Build history of the part. All positions in model axes, mm. Face numbers are marked on the shaded views. Round coordinates to 2 decimals unless told otherwise and drop trailing zeros. Write each loop counter-clockwise with the first axis right and the second up, starting at its lowest first coordinate (ties: lowest second). Pieces come first, ordered by that corner, then holes. Notation, with made-up numbers: (-32.5, -17) - (-7.5, -17) arc R15 cw to (-7.5, -1) - close; hole circle Ø7 at (30, 3). An arc over 180 degrees is marked (long way). One line per question, with ' | ' between items.
from build123d import *

# Parameters (mm, degrees)
SKETCH1_W                = 46
SKETCH1_H                = 12
BOSS_EXTRUDE1_DEPTH      = 12
F_7_0_7_DIAMETER_HOLE1_D = 7
M6X1_0_TAPPED_HOLE1_D    = 5


with BuildPart() as part:
    # Sketch1 → Boss-Extrude1 (new body)
    with BuildSketch(Plane(origin=(0, 0, 0), x_dir=(1, 0, 0), z_dir=(0, 1, 0))):
        with Locations((0, 6)):
            Rectangle(SKETCH1_W, SKETCH1_H)
    extrude(amount=BOSS_EXTRUDE1_DEPTH)

    # Ø7.0 (7) Diameter Hole1 (through all)
    with Locations(Plane(origin=(-8.628001273, 12, -9.044925154), x_dir=(1, 0, 0), z_dir=(0, 1, 0))):
        with Locations((25.628001273, -3.044925154), (-8.371998727, -3.044925154)):
            Hole(F_7_0_7_DIAMETER_HOLE1_D / 2)

    # M6x1.0 Tapped Hole1 (through all)
    with Locations(Plane.XY):
        with Locations((0, 6)):
            Hole(M6X1_0_TAPPED_HOLE1_D / 2)


solid = part.part
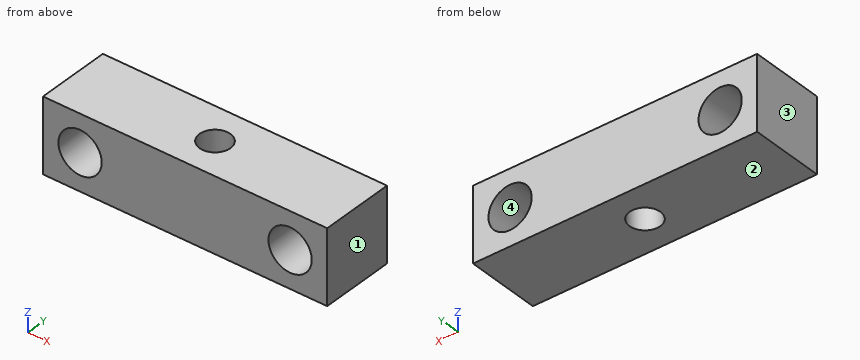
Q1. Drill centre lines: L1, parallel to Z at x = 17, y = 7.5; L2, parallel to Y at x = 0, z = -7.5; L3, parallel to X at y = 7.5, z = -8. Where is each one in solid material? Low to high. Write a range as from..to.
Found:
L1: -12..-9.5, -2.5..0 | L2: 0..3.5, 8.5..12 | L3: -23..-19.87, -14.13..-2, 2..14.13, 19.87..23
Q2. Pull direction X, two halves, no side cores. Call the marked faces 1, 2, 3 and 4: +X half, -X half, draft (parallel to the pull), parting line (faces both ways), or undercut.
Found:
face 1: +X half | face 2: draft | face 3: -X half | face 4: undercut
Q3. Saw through at A-A, the plane z = -6. List the corners of the cut face in (x, y), then the cut area to 3 significant figures.
Found:
outline: (-23, 0) - (-20.5, 0) - (-20.5, 12) - (-23, 12) - close; (-13.5, 0) - (13.5, 0) - (13.5, 12) - (-13.5, 12) - close; (20.5, 0) - (23, 0) - (23, 12) - (20.5, 12) - close; hole circle Ø5 at (0, 6) | area: 364 mm^2
Q4. Drop a flat-ended pin along its axis: pin 1 (5.5 mm diameter, centred on x = -17, z = -6, fed in from +Y). Give the stop position or say it passes through.
Found:
pin 1: through
Q5. Saw through at B-B, the plane y = 6. List the corners of the cut face in (x, z).
Found:
outline: (-23, -12) - (-2.5, -12) - (-2.5, 0) - (-23, 0) - close; (2.5, -12) - (23, -12) - (23, 0) - (2.5, 0) - close; hole circle Ø7 at (-17, -6); hole circle Ø7 at (17, -6)
Q6. Saw through at D-D, the plane z = -11. List the corners of the cut face in (x, y).
Found:
outline: (-23, 0) - (23, 0) - (23, 12) - (-23, 12) - close; hole circle Ø5 at (0, 6)
Q7. Saw through at C-C, the plane x = 0. List the corners of the cut face in (y, z).
Found:
outline: (0, -12) - (3.5, -12) - (3.5, 0) - (0, 0) - close; (8.5, -12) - (12, -12) - (12, 0) - (8.5, 0) - close
